Print and shaded views of the part. All mm, measured from the part's lowest x, y and z. A direction names the side the tool comes from. Give positions to 0.01 mm unless a question says otherwise; leave off trailing zeros. Loops run counter-clockwise (first coordinate to the right, second up) from the corner with the lowest first, then second, coordinate; pieces in that order, holes last. Notation, with made-up numbers: (-7, 82.25) - (15, 82.25) arc R21 cw to (15, 111.25) - close; hole circle Ø1 at (37.5, 71.5). An arc over 180 degrees is marked (long way). Return JSON: item names as keys, results as strings.
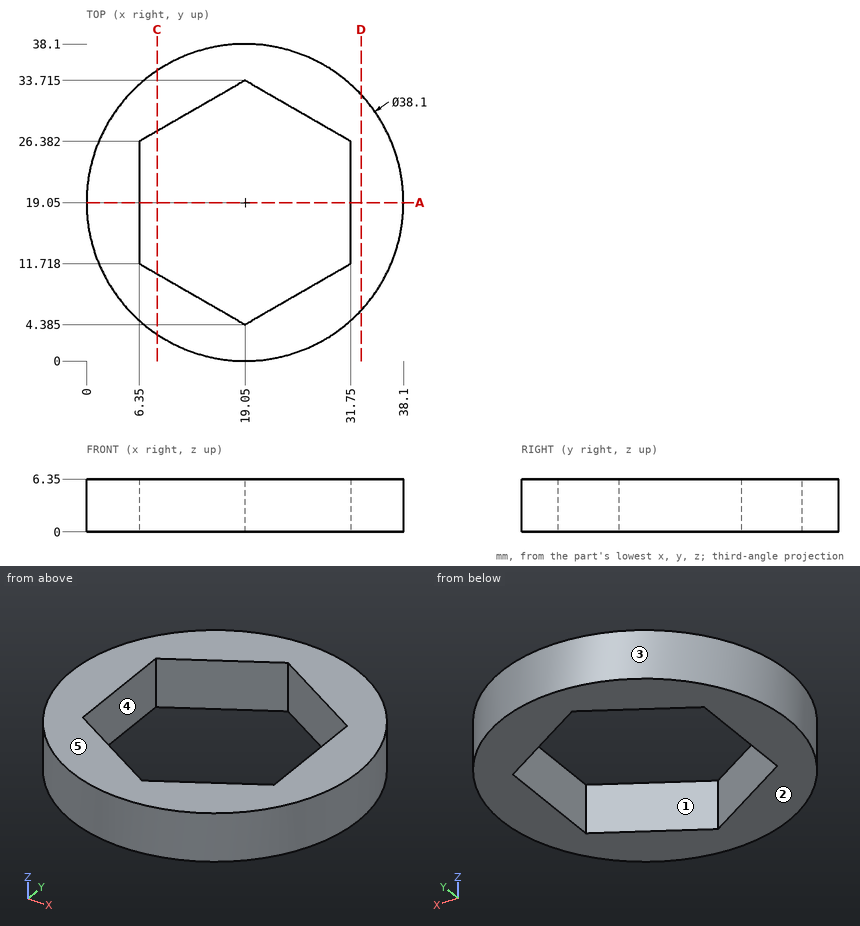
1. Cut at C-C, the plane x = 8.5. Write the cut outline in (y, z).
Values follow:
{"outline": "(3.19, 0) - (10.48, 0) - (10.48, 6.35) - (3.19, 6.35) - close; (27.62, 0) - (34.91, 0) - (34.91, 6.35) - (27.62, 6.35) - close"}
2. Cut at D-D, the plane x = 33. Write the cut outline in (y, z).
Values follow:
{"outline": "(6.08, 0) - (32.02, 0) - (32.02, 6.35) - (6.08, 6.35) - close"}
3. Pull direction X, two halves, no side cores. Call the marked faces 3, 4 and 5: +X half, -X half, draft (parallel to the pull), parting line (faces both ways), or undercut.
Values follow:
{"face 3": "parting line", "face 4": "undercut", "face 5": "draft"}
4. Cut at A-A, the plane y = 19.05. Write the cut outline in (x, z).
Values follow:
{"outline": "(0, 0) - (6.35, 0) - (6.35, 6.35) - (0, 6.35) - close; (31.75, 0) - (38.1, 0) - (38.1, 6.35) - (31.75, 6.35) - close"}
5. Drill centre lines: probe 1 along Y at (x, z) = (24.5, 1.5) (1 decimal); probe 2 along Y at (x, z) = (20, 5.5) (1 decimal); probe 3 along X at (y, z) = (23.5, 2.75). Where is each one in solid material? Low to high.
Values follow:
{"probe 1": "y = 0.8 to 7.5, 30.6 to 37.3", "probe 2": "y = 0 to 4.9, 33.2 to 38.1", "probe 3": "x = 0.53 to 6.35, 31.75 to 37.57"}
6. Drop flat-ended pins along their axis: P1, Ø1.5, axis at y = 28.5, z = 4, coming from the +X side; P2, Ø3, axis at y = 21.5, z = 2, coming from the -X side; P3, Ø2, axis at x = 8, z = 2, coming from the -Y side. Give the stop position or say it passes through.
Values follow:
{"P1": "stops at x = 36", "P2": "stops at x = 0.02", "P3": "stops at y = 2.87"}
7. Which spindle directions (+Z, -Z, +X, -X, +Y, -Y) get a long thin tool onto all of the face, cutting with end or side? Do the marked faces 1 and 2. Say none if no direction does.
Values follow:
{"face 1": "+Z, -Z", "face 2": "-Z, +X, -X, +Y, -Y"}
